Could you check a few things on this model? Use its own coordinates, in mm. A direction names the side the tool comes from. Give positions to 0.01 mm unless a question says otherwise; leave off trailing zeros. Write each loop counter-clockwise with the first axis right and the second up, starting at its lowest first coordinate (ties: lowest second). Pieces come first, ordered by that corner, then holes. Notation, with made-up numbers: (8.5, 44.25) - (60.5, 44.25) arc R13 cw to (60.5, 68.25) - close; hole circle Ø9 at (-6.5, 46.5). An arc over 180 degrees is marked (long way). Answer in a Markdown table with one row per item.
from build123d import *

# Parameters (mm, degrees)
SKETCH_1_W          = 95
SKETCH_1_H          = 95
EXTRUDE_1_DEPTH     = 19
CHAMFER_1_SIZE      = 19
SKETCH_2_R          = 9
CUT_EXTRUDE_1_DEPTH = 5


with BuildPart() as part:
    # Эскиз1 → Бобышка-Вытянуть1 (new body)
    with BuildSketch(Plane.XY):
        Rectangle(SKETCH_1_W, SKETCH_1_H)
    extrude(amount=EXTRUDE_1_DEPTH)

    # Фаска1
    chamfer_1_edges = [part.edges().sort_by_distance(p)[0] for p in [
        (0, 47.5, 19),
        (47.5, 0, 19),
        (0, -47.5, 19),
        (-47.5, 0, 19),
    ]]
    chamfer(chamfer_1_edges, length=CHAMFER_1_SIZE - 0.0001)  # a hair under: the kernel refuses the full size

    # Эскиз2 → Вырез-Вытянуть1 (cut)
    with BuildSketch(Plane.XY.offset(19)):
        Circle(SKETCH_2_R)
        with Locations((19, 0)):
            Circle(SKETCH_2_R)
        with Locations((19, 19)):
            Circle(SKETCH_2_R)
        with Locations((0, 19)):
            Circle(SKETCH_2_R)
        with Locations((-19, 19)):
            Circle(SKETCH_2_R)
        with Locations((-19, 0)):
            Circle(SKETCH_2_R)
        with Locations((-19, -19)):
            Circle(SKETCH_2_R)
        with Locations((0, -19)):
            Circle(SKETCH_2_R)
        with Locations((19, -19)):
            Circle(SKETCH_2_R)
    extrude(amount=-CUT_EXTRUDE_1_DEPTH, mode=Mode.SUBTRACT)


solid = part.part
1) Imagine slicing it at C-C (z = 16.75). State how many separate pieces and enclosed holes the cut face has, then the cut area to 3 significant figures.
Check values:
| item | result |
|---|---|
| separate pieces | 1 |
| enclosed holes | 9 |
| area | 1,490 mm2 |
2) On a 3-axis mill with a long thin cutter (end or side, diameter ignored), from which of +Z, -Z, +X, -X, +Y, -Y can I reach the whole of each face in a straight line? I mean faces 1 (the face through (-1.172, -10.077, 16.535)), 2 (the face through (-0.7, -37.9, 9.6)). Say none if no direction works.
Check values:
| item | result |
|---|---|
| face 1 | +Z |
| face 2 | +Z, +X, -X, -Y |
3) Will these pins go through, and if not, where does the flat tip stop? P1, Ø20.5, axis at x = 19, y = 0, coming from the -Z side; P2, Ø5.5, axis at x = -22, y = 3, coming from the +Z side; P3, Ø10, axis at y = 34.5, z = 10, coming from the -X side; P4, Ø5, axis at x = -26.5, z = 4.5, coming from the +Y side.
Check values:
| item | result |
|---|---|
| P1 | stops at z = 0 |
| P2 | stops at z = 14 |
| P3 | stops at x = -42.5 |
| P4 | stops at y = 45.5 |
4) Imagine slicing it at D-D (z = 7). List the corners of the cut face in (x, y) for me, then the cut area to 3 significant figures.
Check values:
| item | result |
|---|---|
| outline | (-40.5, -40.5) - (40.5, -40.5) - (40.5, 40.5) - (-40.5, 40.5) - close |
| area | 6,560 mm2 |
5) We'd pull the mould along Y, two halves only. Please class faces 3 (the face through (-0.7, 37.9, 9.6)), 4 (the face through (27.584, 2.703, 16.535)), 5 (the face through (37.9, -0.7, 9.6)): +Y half, -Y half, draft (parallel to the pull), parting line (faces both ways), or undercut.
Check values:
| item | result |
|---|---|
| face 3 | +Y half |
| face 4 | undercut |
| face 5 | draft |
6) If I drill on line 1 (Y direction, x = 19, z = 15.9); line 2 (Y direction, x = 19, z = 17.5); line 3 (Z direction, x = -17.5, y = 5), over which ranges is the centre line in solid material (lowest first)?
Check values:
| item | result |
|---|---|
| line 1 | y = -31.6 to -28, -10 to -9, 9 to 10, 28 to 31.6 |
| line 2 | y = -30 to -28, -10 to -9, 9 to 10, 28 to 30 |
| line 3 | z = 0 to 14 |
